Design review of the part shown in the three views and the two pictorial views. Dimensions are in mm from the part's minimum x, y and z. Round coordinates to 2 decimals unless told otherwise and drop trailing zeros. Order: outer loops, then holes, each group sorted by start corner. A loop starts at its lowest first (then second) coordinate and runs counter-clockwise, first axis right, second up.
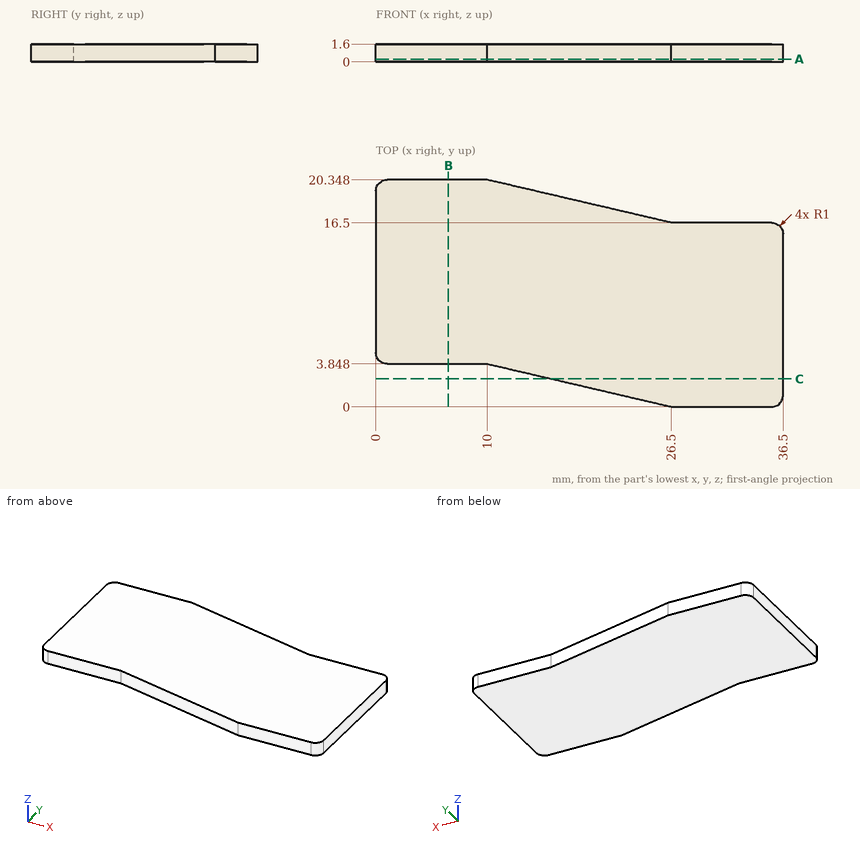
(1) Consider section A-A (z = 0.25). Write out the cut boundary in (x, y), and give its area (3 significant figures).
Data:
outline: (0, 4.85) arc R1 ccw to (1, 3.85) - (10, 3.85) - (26.5, 0) - (35.5, 0) arc R1 ccw to (36.5, 1) - (36.5, 15.5) arc R1 ccw to (35.5, 16.5) - (26.5, 16.5) - (10, 20.35) - (1, 20.35) arc R1 ccw to (0, 19.35) - close
area: 601 mm2
(2) Insertion check: pin 1 (0.5 mm diameter, centred on x = 30.5, z = 0.5, fed in from +Y). The pin has a flat end and moves straight along its axis. Give the tip position at first contact, or say it passes through.
Data:
pin 1: stops at y = 16.5
(3) To check wall thickness, follow probe 1 along Y at (x, z) = (34.5, 0.3); probe 2 along Y at (x, z) = (8.5, 0.6); probe 3 along X at (y, z) = (4.5, 1.1). State the ranges of each line that lie inside material, in increasing order.
Data:
probe 1: y = 0 to 16.5
probe 2: y = 3.85 to 20.35
probe 3: x = 0.06 to 36.5
(4) Consider section C-C (y = 2.5). Write out the cut boundary in (x, z).
Data:
outline: (15.78, 0) - (36.5, 0) - (36.5, 1.6) - (15.78, 1.6) - close
(5) Consider section B-B (x = 6.5). Write out the cut boundary in (y, z), and give its area (3 significant figures).
Data:
outline: (3.85, 0) - (20.35, 0) - (20.35, 1.6) - (3.85, 1.6) - close
area: 26.4 mm2
